from build123d import *

# Parameters (mm, degrees)
SKETCH_1_W          = 130
SKETCH_1_H          = 130
SKETCH_1_R          = 22.5
EXTRUDE_1_DEPTH     = 3
FILLET_1_R          = 35
SKETCH_5_R          = 2
SKETCH_5_W          = 15
SKETCH_5_H          = 15
CUT_EXTRUDE_2_DEPTH = 13
SKETCH_6_R          = 1.5
CUT_EXTRUDE_3_DEPTH = 92.972822073
SKETCH_7_R          = 1.5
CUT_EXTRUDE_4_DEPTH = 92.972822073


with BuildPart() as part:
    # 草图1 → 凸台-拉伸1 (new body)
    with BuildSketch(Plane.XY):
        Rectangle(SKETCH_1_W, SKETCH_1_H)
        Circle(SKETCH_1_R, mode=Mode.SUBTRACT)
    extrude(amount=-EXTRUDE_1_DEPTH)

    # 圆角1
    fillet_1_edges = [part.edges().sort_by_distance(p)[0] for p in [
        (65, -65, -1.5),
        (-65, -65, -1.5),
        (-65, 65, -1.5),
        (65, 65, -1.5),
    ]]
    fillet(fillet_1_edges, radius=FILLET_1_R)

    # 草图5 → 切除-拉伸2 (cut)
    with BuildSketch(Plane(origin=(0, 0, -3), x_dir=(-1, 0, 0), z_dir=(0, 0, -1))):
        with Locations((36.119111303, 58.196758832)):
            Circle(SKETCH_5_R)
        with Locations((36.119111303, 48.196758832)):
            Circle(SKETCH_5_R)
        with Locations((36.119111303, 38.196758832)):
            Circle(SKETCH_5_R)
        with Locations((-36.119111303, -58.196758832)):
            Circle(SKETCH_5_R)
        with Locations((16.119111303, 48.196758832)):
            Circle(SKETCH_5_R)
        with Locations((16.119111303, 38.196758832)):
            Circle(SKETCH_5_R)
        with Locations((16.119111303, 28.196758832)):
            Circle(SKETCH_5_R)
        with Locations((26.119111303, 58.196758832)):
            Circle(SKETCH_5_R)
        with Locations((16.119111303, -48.196758832)):
            Circle(SKETCH_5_R)
        with Locations((26.119111303, -28.196758832)):
            Circle(SKETCH_5_R)
        with Locations((36.119111303, 28.196758832)):
            Circle(SKETCH_5_R)
        with Locations((26.119111303, 48.196758832)):
            Circle(SKETCH_5_R)
        with Locations((26.119111303, 38.196758832)):
            Circle(SKETCH_5_R)
        with Locations((26.119111303, 28.196758832)):
            Circle(SKETCH_5_R)
        with Locations((16.119111303, 58.196758832)):
            Circle(SKETCH_5_R)
        with Locations((16.119111303, -58.196758832)):
            Circle(SKETCH_5_R)
        with Locations((26.119111303, -58.196758832)):
            Circle(SKETCH_5_R)
        with Locations((16.119111303, -28.196758832)):
            Circle(SKETCH_5_R)
        with Locations((16.119111303, -38.196758832)):
            Circle(SKETCH_5_R)
        with Locations((36.119111303, -38.196758832)):
            Circle(SKETCH_5_R)
        with Locations((36.119111303, -48.196758832)):
            Circle(SKETCH_5_R)
        with Locations((36.119111303, -58.196758832)):
            Circle(SKETCH_5_R)
        with Locations((-36.119111303, -48.196758832)):
            Circle(SKETCH_5_R)
        with Locations((-36.119111303, -38.196758832)):
            Circle(SKETCH_5_R)
        with Locations((-16.119111303, -38.196758832)):
            Circle(SKETCH_5_R)
        with Locations((-16.119111303, -28.196758832)):
            Circle(SKETCH_5_R)
        with Locations((-26.119111303, -58.196758832)):
            Circle(SKETCH_5_R)
        with Locations((26.119111303, -38.196758832)):
            Circle(SKETCH_5_R)
        with Locations((26.119111303, -48.196758832)):
            Circle(SKETCH_5_R)
        with Locations((36.119111303, -28.196758832)):
            Circle(SKETCH_5_R)
        with Locations((-36.119111303, -28.196758832)):
            Circle(SKETCH_5_R)
        with Locations((-26.119111303, -48.196758832)):
            Circle(SKETCH_5_R)
        with Locations((-26.119111303, -38.196758832)):
            Circle(SKETCH_5_R)
        with Locations((-26.119111303, -28.196758832)):
            Circle(SKETCH_5_R)
        with Locations((-16.119111303, -48.196758832)):
            Circle(SKETCH_5_R)
        with Locations((-16.119111303, 28.196758832)):
            Circle(SKETCH_5_R)
        with Locations((-16.119111303, 38.196758832)):
            Circle(SKETCH_5_R)
        with Locations((-16.119111303, 48.196758832)):
            Circle(SKETCH_5_R)
        with Locations((-26.119111303, 28.196758832)):
            Circle(SKETCH_5_R)
        with Locations((-26.119111303, 38.196758832)):
            Circle(SKETCH_5_R)
        with Locations((-36.119111303, 38.196758832)):
            Circle(SKETCH_5_R)
        with Locations((-36.119111303, 48.196758832)):
            Circle(SKETCH_5_R)
        with Locations((-36.119111303, 58.196758832)):
            Circle(SKETCH_5_R)
        with Locations((-16.119111303, -58.196758832)):
            Circle(SKETCH_5_R)
        with Locations((-16.119111303, 58.196758832)):
            Circle(SKETCH_5_R)
        with Locations((-26.119111303, 58.196758832)):
            Circle(SKETCH_5_R)
        with Locations((-26.119111303, 48.196758832)):
            Circle(SKETCH_5_R)
        with Locations((-36.119111303, 28.196758832)):
            Circle(SKETCH_5_R)
        with Locations((35.031984266, -1.155156202)):
            Rectangle(SKETCH_5_W, SKETCH_5_H)
        with Locations((-35.031984266, -1.155156202)):
            Rectangle(SKETCH_5_W, SKETCH_5_H)
    extrude(amount=-CUT_EXTRUDE_2_DEPTH, mode=Mode.SUBTRACT)

    # 草图6 → 切除-拉伸3 (cut, through all)
    with BuildSketch(Plane.XY):
        with Locations((-45, 20)):
            Circle(SKETCH_6_R)
        with Locations((45, 20)):
            Circle(SKETCH_6_R)
        with Locations((45, -20)):
            Circle(SKETCH_6_R)
        with Locations((-45, -20)):
            Circle(SKETCH_6_R)
    extrude(amount=-CUT_EXTRUDE_3_DEPTH, mode=Mode.SUBTRACT)

    # 草图7 → 切除-拉伸4 (cut, through all)
    with BuildSketch(Plane.XY):
        with Locations((-20, 45)):
            Circle(SKETCH_7_R)
        with Locations((20, 45)):
            Circle(SKETCH_7_R)
        with Locations((20, -45)):
            Circle(SKETCH_7_R)
        with Locations((-20, -45)):
            Circle(SKETCH_7_R)
    extrude(amount=-CUT_EXTRUDE_4_DEPTH, mode=Mode.SUBTRACT)


solid = part.part
Work out the finished part from the listing and answer in its coordinate system (mm). Coordinates: 2 decimals unless noted, no trailing zeros. Loops run counter-clockwise (first coordinate to the right, second up) from the corner with the lowest first, then second, coordinate; pieces in that order, holes last. Notation, with made-up numbers: (68.5, 0) -> (115.5, 0) arc R21 ccw to (115.5, 14) -> close; hole circle Ø6 at (-12.5, -6.75). An arc over 180 degrees is marked (long way). Write each question's results on one line, items separated by ' | '. Start each with the question number.
1) Consider line 1 along Y through (x, z) = (-1, -1.05); line 2 along X through (y, z) = (46, -0.6); line 3 along Y through (x, z) = (13.5, -2.5). Determine where each line is inside the solid, lowest interval first.
2) Find section A-A on x = 0. Determine the outline of the cut face in (y, z), then the cut area to 3 significant figures.
3) The mould has two halves that part along X. Classify faces 1 (the cylindrical face through (-55.019, -54.475, -1.521)), 2 (the cylindrical face through (25.2, 56.42, -1.52)), 3 (the flat face through (27.532, -1, -2)), 4 (the flat face through (-1, -28, 0)): pulls with the +X half, pulls with the -X half, needs draft (parallel to the pull), parting line crosses it, or undercut.
4) Find section C-C on x = -20. Determine the outline of the cut face in (y, z).
5) Find section D-D on x = -45. Determine the outline of the cut face in (y, z).
6) Find section B-B on y = 0. Determine the outline of the cut face in (x, z), then the cut area to 3 significant figures.
7) Flat-ended cylindrical pins translate along their axes: P1, Ø1.5, axis at y = -32, z = -2, coming from the -X side; P2, Ø4.5, axis at x = -26.12, y = 58.2, coming from the +Z side; P3, Ø3.5, axis at x = 36.12, y = 28.2, coming from the -Z side; P4, Ø1.5, axis at x = 33, z = -1.5, coming from the -Y side. Find the tip coordinate at first contact, or state that the pin passes through.
Response values:
1) line 1: y = -65 to -22.48, 22.48 to 65 | line 2: x = -61.13 to -21.12, -18.88 to 18.88, 21.12 to 61.13 | line 3: y = -65 to -18, 18 to 65
2) outline: (-65, -3) -> (-22.5, -3) -> (-22.5, 0) -> (-65, 0) -> close; (22.5, -3) -> (65, -3) -> (65, 0) -> (22.5, 0) -> close | area: 255 mm^2
3) face 1: pulls with the -X half | face 2: undercut | face 3: undercut | face 4: needs draft
4) outline: (-65, -3) -> (-46.5, -3) -> (-46.5, 0) -> (-65, 0) -> close; (-43.5, -3) -> (-10.31, -3) -> (-10.31, 0) -> (-43.5, 0) -> close; (10.31, -3) -> (43.5, -3) -> (43.5, 0) -> (10.31, 0) -> close; (46.5, -3) -> (65, -3) -> (65, 0) -> (46.5, 0) -> close
5) outline: (-61.62, -3) -> (-21.5, -3) -> (-21.5, 0) -> (-61.62, 0) -> close; (-18.5, -3) -> (18.5, -3) -> (18.5, 0) -> (-18.5, 0) -> close; (21.5, -3) -> (61.62, -3) -> (61.62, 0) -> (21.5, 0) -> close
6) outline: (-65, -3) -> (-42.53, -3) -> (-42.53, 0) -> (-65, 0) -> close; (-27.53, -3) -> (-22.5, -3) -> (-22.5, 0) -> (-27.53, 0) -> close; (22.5, -3) -> (27.53, -3) -> (27.53, 0) -> (22.5, 0) -> close; (42.53, -3) -> (65, -3) -> (65, 0) -> (42.53, 0) -> close | area: 165 mm^2
7) P1: stops at x = -64.98 | P2: stops at z = 0 | P3: passes through | P4: stops at y = -64.93
